Build history of the part. All positions in model axes, mm. Face numbers are marked on the shaded views. A direction names the side the tool comes from. Coordinates: 2 decimals unless noted, no trailing zeros. Loops run counter-clockwise (first coordinate to the right, second up) from the corner with the lowest first, then second, coordinate; pieces in that order, holes last.
(1) Tool access for the marked faces 4 and 5: list every direction of +Z, -Z, +X, -X, +Y, -Y with a clear straight run to the whole face (end or side of a thin tool).
(2) Wall check: L1, parallel to X at y = -13.5, z = 11.43; L2, parallel to Y at x = -8.5, z = 13.5; L3, parallel to Z at x = 13.25, y = 2. Give the ranges that are in metal, low to high.
(3) Flat gauge pins, fed straight in: P1, Ø5.5, axis at x = 0, z = 16.5, coming from the +Y side; P2, Ø8, axis at y = -1.27, z = 10.922, coming from the -X side; P3, Ø5, axis at y = -11, z = 17, coming from the -X side. Where does each tip first touch, or does it go through?
(4) Two-plate mould, pull along Y, no slides. Class the marked faces 1, 2 and 3: pulls with the +Y half, pulls with the -Y half, needs draft (parallel to the pull), parting line crosses it, or undercut.
(5) Slice it at A-A (x = 1.27). Give the cut face in (y, z), and give its area (3 significant figures).
(6) Slice it at D-D (z = 10.75). Give the number of separate pieces and of enclosed holes in the cut face, and give its area (3 significant figures).
(7) Slice it at B-B (y = -1.27). Give the cut face in (x, z).
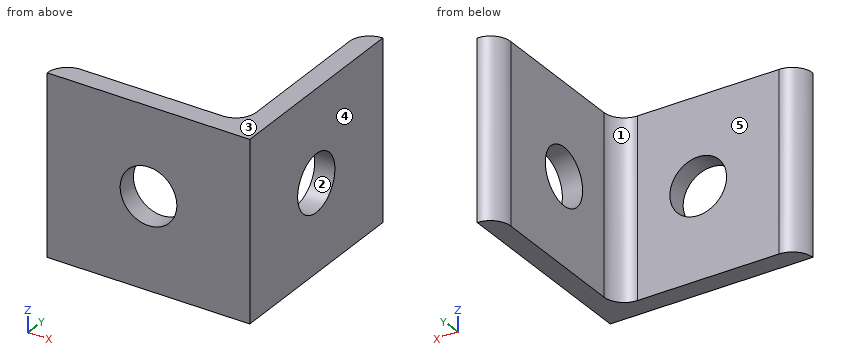
from build123d import *

# Parameters (mm, degrees)
EXTRUDE_THIN1_DEPTH = 22.352
FILLET1_R           = 2.54
SKETCH2_R           = 3.556
CUT_EXTRUDE1_DEPTH  = 2.54
SKETCH3_R           = 3.556
CUT_EXTRUDE2_DEPTH  = 2.54


with BuildPart() as part:
    # Sketch1 → Extrude-Thin1 (new body)
    with BuildSketch(Plane.XY):
        Polygon((-11.43, -11.43), (11.43, -11.43), (11.43, 11.43), (13.97, 11.43), (13.97, -13.97), (-11.43, -13.97), align=None)
    extrude(amount=EXTRUDE_THIN1_DEPTH)

    # Fillet1
    fillet1_edges = [part.edges().sort_by_distance(p)[0] for p in [
        (11.43, 11.43, 11.176),
        (-11.43, -11.43, 11.176),
        (11.43, -11.43, 11.176),
    ]]
    fillet(fillet1_edges, radius=FILLET1_R - 0.0001)  # a hair under: the kernel refuses the full size

    # Sketch2 → Cut-Extrude1 (cut)
    with BuildSketch(Plane.XZ.offset(13.97)):
        with Locations(Location((1.27, 11.43, 0), (0, 0, 270))):
            Circle(SKETCH2_R)
    extrude(amount=-CUT_EXTRUDE1_DEPTH, mode=Mode.SUBTRACT)

    # Sketch3 → Cut-Extrude2 (cut)
    with BuildSketch(Plane(origin=(13.97, 0, 0), x_dir=(0, 0, -1), z_dir=(1, 0, 0))):
        with Locations((-10.922, -1.27)):
            Circle(SKETCH3_R)
    extrude(amount=-CUT_EXTRUDE2_DEPTH, mode=Mode.SUBTRACT)


solid = part.part
Response values:
1. face 4: +Z, -Z, +X, +Y, -Y
1. face 5: +Z, -Z, -X, +Y
2. L1: x = -11.39 to -2.29, 4.83 to 13.97
2. L2: y = -13.97 to -11.43
2. L3: z = 0 to 9.52, 12.32 to 22.35
3. P1: stops at y = -11.43
3. P2: stops at x = 11.43
3. P3: stops at x = -11.39
4. face 1: pulls with the +Y half
4. face 2: undercut
4. face 3: needs draft
5. outline: (-13.97, 0) - (-11.43, 0) - (-11.43, 7.87) - (-13.97, 7.87) - close; (-13.97, 14.99) - (-11.43, 14.99) - (-11.43, 22.35) - (-13.97, 22.35) - close
5. area: 38.7 mm2
6. separate pieces: 3
6. enclosed holes: 0
6. area: 85.4 mm2
7. outline: (11.43, 0) - (13.97, 0) - (13.97, 7.37) - (11.43, 7.37) - close; (11.43, 14.48) - (13.97, 14.48) - (13.97, 22.35) - (11.43, 22.35) - close
